Could you check a few things on this model? Use its own coordinates, in mm. A direction names the side the tool comes from. Coordinates: 2 decimals unless noted, no trailing zeros. Write each loop counter-clockwise with the first axis right and the second up, starting at its lowest first coordinate (ties: lowest second). Pieces come first, ordered by that corner, then holes.
```python
from build123d import *

# Parameters (mm, degrees)
SKETCH1_W                                           = 65
SKETCH1_H                                           = 65
BOSS_EXTRUDE1_DEPTH                                 = 12
SKETCH3_R                                           = 12.8
CUT_EXTRUDE1_DEPTH                                  = 12
SKETCH4_W                                           = 5
SKETCH4_H                                           = 40
CUT_EXTRUDE2_DEPTH                                  = 12
SKETCH5_W                                           = 10
SKETCH5_H                                           = 13
BOSS_EXTRUDE4_DEPTH                                 = 12
LPATTERN1_COUNT                                     = 2
LPATTERN1_PITCH                                     = 15
CBORE_FOR_M6_HEX_SOCKET_HEAD_CAP_SCREW1_D           = 6.6
CBORE_FOR_M6_HEX_SOCKET_HEAD_CAP_SCREW1_CBORE_D     = 10.5
CBORE_FOR_M6_HEX_SOCKET_HEAD_CAP_SCREW1_CBORE_DEPTH = 6.75
CUT_EXTRUDE3_DEPTH                                  = 5.1
CBORE_FOR_M6_HEX_SOCKET_HEAD_CAP_SCREW2_D           = 7.5
CBORE_FOR_M6_HEX_SOCKET_HEAD_CAP_SCREW2_CBORE_D     = 11.4
CBORE_FOR_M6_HEX_SOCKET_HEAD_CAP_SCREW2_CBORE_DEPTH = 6.75
CBORE_FOR_M6_HEX_SOCKET_HEAD_CAP_SCREW3_D           = 7.5
CBORE_FOR_M6_HEX_SOCKET_HEAD_CAP_SCREW3_CBORE_D     = 11.4
CBORE_FOR_M6_HEX_SOCKET_HEAD_CAP_SCREW3_CBORE_DEPTH = 6.75
CBORE_FOR_M6_HEX_SOCKET_HEAD_CAP_SCREW4_D           = 7.5
CBORE_FOR_M6_HEX_SOCKET_HEAD_CAP_SCREW4_CBORE_D     = 11.4
CBORE_FOR_M6_HEX_SOCKET_HEAD_CAP_SCREW4_CBORE_DEPTH = 6.75
CBORE_FOR_M6_HEX_SOCKET_HEAD_CAP_SCREW5_D           = 7.5
CBORE_FOR_M6_HEX_SOCKET_HEAD_CAP_SCREW5_CBORE_D     = 11.4
CBORE_FOR_M6_HEX_SOCKET_HEAD_CAP_SCREW5_CBORE_DEPTH = 6.75


with BuildPart() as part:
    # Sketch1 → Boss-Extrude1 (new body)
    with BuildSketch(Plane(origin=(0, 0, 0), x_dir=(1, 0, 0), z_dir=(0, 1, 0))):
        Rectangle(SKETCH1_W, SKETCH1_H)
    extrude(amount=BOSS_EXTRUDE1_DEPTH)

    # Sketch3 → Cut-Extrude1 (cut)
    with BuildSketch(Plane(origin=(0, 12, 0), x_dir=(-1, 0, 0), z_dir=(0, 1, 0))):
        with Locations(Location((0, 0, 0), (0, 0, 90))):
            Circle(SKETCH3_R)
    extrude(amount=-CUT_EXTRUDE1_DEPTH, mode=Mode.SUBTRACT)

    # Sketch4 → Cut-Extrude2 (cut)
    with BuildSketch(Plane(origin=(0, 12, 0), x_dir=(-1, 0, 0), z_dir=(0, 1, 0))):
        with Locations((0, -32.5)):
            Rectangle(SKETCH4_W, SKETCH4_H)
    extrude(amount=-CUT_EXTRUDE2_DEPTH, mode=Mode.SUBTRACT)

    # Sketch5 → Boss-Extrude4 (add)
    with BuildSketch(Plane(origin=(0, 12, 0), x_dir=(-1, 0, 0), z_dir=(0, 1, 0))):
        with Locations((7.5, -39)):
            Rectangle(SKETCH5_W, SKETCH5_H)
    boss_extrude4 = extrude(amount=-BOSS_EXTRUDE4_DEPTH)

    # LPattern1: Boss-Extrude4 ×2
    with Locations(*[(i * LPATTERN1_PITCH, 0, 0) for i in range(1, LPATTERN1_COUNT)]):
        add(boss_extrude4)

    # CBORE for M6 Hex Socket Head Cap Screw1 (through all)
    with Locations(Plane.ZY.offset(12.5)):
        with Locations((-39, 6)):
            CounterBoreHole(CBORE_FOR_M6_HEX_SOCKET_HEAD_CAP_SCREW1_D / 2, CBORE_FOR_M6_HEX_SOCKET_HEAD_CAP_SCREW1_CBORE_D / 2, CBORE_FOR_M6_HEX_SOCKET_HEAD_CAP_SCREW1_CBORE_DEPTH)

    # Sketch9 → Cut-Extrude3 (cut)
    with BuildSketch(Plane(origin=(12.5, 0, 0), x_dir=(0, 0, -1), z_dir=(1, 0, 0))):
        Polygon((44.773502692, 6), (41.886751346, 11), (36.113248654, 11), (33.226497308, 6), (36.113248654, 1), (41.886751346, 1), align=None)
    extrude(amount=-CUT_EXTRUDE3_DEPTH, mode=Mode.SUBTRACT)

    # CBORE for M6 Hex Socket Head Cap Screw2 (through all)
    with Locations(Plane(origin=(0, 12, 0), x_dir=(-1, 0, 0), z_dir=(0, 1, 0))):
        with Locations((25, -25)):
            CounterBoreHole(CBORE_FOR_M6_HEX_SOCKET_HEAD_CAP_SCREW2_D / 2, CBORE_FOR_M6_HEX_SOCKET_HEAD_CAP_SCREW2_CBORE_D / 2, CBORE_FOR_M6_HEX_SOCKET_HEAD_CAP_SCREW2_CBORE_DEPTH)

    # CBORE for M6 Hex Socket Head Cap Screw3 (through all)
    with Locations(Plane(origin=(0, 12, 0), x_dir=(-1, 0, 0), z_dir=(0, 1, 0))):
        with Locations((-25, -25)):
            CounterBoreHole(CBORE_FOR_M6_HEX_SOCKET_HEAD_CAP_SCREW3_D / 2, CBORE_FOR_M6_HEX_SOCKET_HEAD_CAP_SCREW3_CBORE_D / 2, CBORE_FOR_M6_HEX_SOCKET_HEAD_CAP_SCREW3_CBORE_DEPTH)

    # CBORE for M6 Hex Socket Head Cap Screw4 (through all)
    with Locations(Plane(origin=(0, 12, 0), x_dir=(-1, 0, 0), z_dir=(0, 1, 0))):
        with Locations((-25, 25)):
            CounterBoreHole(CBORE_FOR_M6_HEX_SOCKET_HEAD_CAP_SCREW4_D / 2, CBORE_FOR_M6_HEX_SOCKET_HEAD_CAP_SCREW4_CBORE_D / 2, CBORE_FOR_M6_HEX_SOCKET_HEAD_CAP_SCREW4_CBORE_DEPTH)

    # CBORE for M6 Hex Socket Head Cap Screw5 (through all)
    with Locations(Plane(origin=(0, 12, 0), x_dir=(-1, 0, 0), z_dir=(0, 1, 0))):
        with Locations((25, 25)):
            CounterBoreHole(CBORE_FOR_M6_HEX_SOCKET_HEAD_CAP_SCREW5_D / 2, CBORE_FOR_M6_HEX_SOCKET_HEAD_CAP_SCREW5_CBORE_D / 2, CBORE_FOR_M6_HEX_SOCKET_HEAD_CAP_SCREW5_CBORE_DEPTH)


solid = part.part
```
1. Please list where these lines run through material, in increasing order: line 1 along Z through (x, y) = (25, 7); line 2 along Z through (x, y) = (8, 6); line 3 along X through (y, z) = (8.75, -37).
Verdict:
line 1: z = -32.5 to -30.7, -19.3 to 19.3, 30.7 to 32.5
line 2: z = -45.5 to -44.77, -33.23 to -9.99, 9.99 to 32.5
line 3: x = -5.75 to -2.5, 2.5 to 7.4
2. I want a section at A-A on z = 0. Please give me the cut outline in (x, y).
Verdict:
outline: (-32.5, 0) - (-12.8, 0) - (-12.8, 12) - (-32.5, 12) - close; (12.8, 0) - (32.5, 0) - (32.5, 12) - (12.8, 12) - close
3. I want a section at B-B on y = 3.75. Give the number of separate pieces and of enclosed holes in the cut face, plus the area to 3 significant figures.
Verdict:
separate pieces: 3
enclosed holes: 4
area: 3,550 mm2
4. On a 3-axis mill with a long thin cutter (end or side, diameter ignored), from which of +Z, -Z, +X, -X, +Y, -Y can I reach the whole of each face in a straight line? I mean faces 1 (the face through (9.986, 8.535, -34.69)), 2 (the face through (-9.17, 9.55, -42.87)), 3 (the face through (-26, 5.25, -29)). Say none if no direction works.
Verdict:
face 1: +X
face 2: -X
face 3: +Y
5. If we mould it in two halves opening along X, with no side actions, what happens to faces 4 (the face through (32.5, 6, 0)), 5 (the face through (9.986, 8.465, -43.35)), 6 (the face through (24, 5.25, 21))? For each: pulls with the +X half, pulls with the -X half, needs draft (parallel to the pull), parting line crosses it, or undercut.
Verdict:
face 4: pulls with the +X half
face 5: needs draft
face 6: undercut
6. For pin 1 (6 mm diameter, centred on x = 19, y = 7, fed in from -Z); pin 2 (9 mm diameter, centred on x = -25, z = 25, fed in from -Y); pin 3 (3.5 mm diameter, centred on x = 26, z = -24, fed in from +Y); pin 4 (9 mm diameter, centred on x = 25, z = 25, fed in from +Y), each with a flat end and sliding along its axis, tell me the tip position at first contact or that it passes through.
Verdict:
pin 1: stops at z = -32.5
pin 2: stops at y = 0
pin 3: passes through
pin 4: stops at y = 5.25
7. I want a section at D-D on x = 9.5. Please give me the cut outline in (y, z), plus the area to 3 significant figures.
Verdict:
outline: (0, -45.5) - (12, -45.5) - (12, -8.58) - (0, -8.58) - close; (0, 8.58) - (12, 8.58) - (12, 32.5) - (0, 32.5) - close; hole (1, -41.89) - (6, -44.77) - (11, -41.89) - (11, -36.11) - (6, -33.23) - (1, -36.11) - close
area: 644 mm2
8. I want a section at C-C on z = 25. Please give me the cut outline in (x, y).
Verdict:
outline: (-32.5, 0) - (-28.75, 0) - (-28.75, 5.25) - (-30.7, 5.25) - (-30.7, 12) - (-32.5, 12) - close; (-21.25, 0) - (21.25, 0) - (21.25, 5.25) - (19.3, 5.25) - (19.3, 12) - (-19.3, 12) - (-19.3, 5.25) - (-21.25, 5.25) - close; (28.75, 0) - (32.5, 0) - (32.5, 12) - (30.7, 12) - (30.7, 5.25) - (28.75, 5.25) - close
